from build123d import *

# Parameters (mm, degrees)
SKETCH2_W                = 45
SKETCH2_H                = 90
EXTRUDE2_DEPTH           = 9.525
SKETCH4_W                = 70
SKETCH4_H                = 9.525
CUT_EXTRUDE1_DEPTH       = 65.348470262
SKETCH5_W                = 8.5
SKETCH5_H                = 70
CUT_EXTRUDE2_DEPTH       = 54.797328001
FILLET1_R                = 6.35
F_6_0_6_DIAMETER_HOLE1_D = 6
M8_CLEARANCE_HOLE1_D     = 9


with BuildPart() as part:
    # Sketch2 → Extrude2 (new, symmetric)
    with BuildSketch(Plane(origin=(0, 0, 0), x_dir=(1, 0, 0), z_dir=(0, 1, 0))):
        Rectangle(SKETCH2_W, SKETCH2_H)
    extrude(amount=EXTRUDE2_DEPTH, both=True)

    # Sketch4 → Cut-Extrude1 (cut, through all)
    with BuildSketch(Plane(origin=(22.5, 0, 0), x_dir=(0, 0, -1), z_dir=(1, 0, 0))):
        with Locations((10, -4.7625)):
            Rectangle(SKETCH4_W, SKETCH4_H)
    extrude(amount=-CUT_EXTRUDE1_DEPTH, mode=Mode.SUBTRACT)

    # Sketch5 → Cut-Extrude2 (cut, through all)
    with BuildSketch(Plane(origin=(0, 9.525, 0), x_dir=(1, 0, 0), z_dir=(0, 1, 0))):
        with Locations((-18.25, 10)):
            Rectangle(SKETCH5_W, SKETCH5_H)
        with Locations((18.25, 10)):
            Rectangle(SKETCH5_W, SKETCH5_H)
    extrude(amount=-CUT_EXTRUDE2_DEPTH, mode=Mode.SUBTRACT)

    # Fillet1
    fillet1_edges = [part.edges().sort_by_distance(p)[0] for p in [
        (-14, 4.7625, 25),
        (14, 4.7625, 25),
    ]]
    fillet(fillet1_edges, radius=FILLET1_R)

    # Ø6.0 (6) Diameter Hole1 (through all)
    with Locations(Plane(origin=(0, 9.525, 0), x_dir=(-1, 0, 0), z_dir=(0, 1, 0))):
        with Locations((-8, -12.5), (8, -12.5)):
            Hole(F_6_0_6_DIAMETER_HOLE1_D / 2)

    # M8 Clearance Hole1 (through all)
    with Locations(Plane(origin=(0, 9.525, 0), x_dir=(-1, 0, 0), z_dir=(0, 1, 0))):
        with Locations((0, -27.5), (0, 2.5)):
            Hole(M8_CLEARANCE_HOLE1_D / 2)


solid = part.part
Geometry: final body of the model. Coordinates: model frame, mm. A direction names the side the tool comes from. Round coordinates to 2 decimals unless told otherwise and drop trailing zeros. Loops run counter-clockwise (first coordinate to the right, second up) from the corner with the lowest first, then second, coordinate; pieces in that order, holes last. Notation, with made-up numbers: M 44.5,46 L 94.5,46 A29 cw 94.5,80 Z; hole C 5,-20 d6. An arc over 180 degrees is marked long. One line per question, with ' | ' between items.
(1) Access query for faces 1 (the flat face through (-14, 5, -13)), 2 (the flat face through (14, 5, -13)), 3 (the flat face through (0, 0, -10)). Directions: +Z, -Z, +X, -X, +Y, -Y. A direction counts if a zero-diameter tool reaches every point of the face in a straight line with its end or side. Return the directions, or none.
Check result:
face 1: -Z, -X, +Y, -Y | face 2: -Z, +X, +Y, -Y | face 3: -Z, +X, -X, -Y
(2) Pull-direction query (Z, two-part tool) for faces 4 (the cylindrical face through (10.77, 4.7, -13.65)), 5 (the cylindrical face through (-15.81, 4.7, 23.09)), 6 (the flat face through (-22.5, 0, 35)); classes: +Z half, -Z half, draft (parallel to the pull), parting line (faces both ways), or undercut.
Check result:
face 4: undercut | face 5: -Z half | face 6: draft
(3) Cut plane A-A on x = 0. Return the cut outline in (y, z) (3 decimals).
Check result:
outline: M -9.525,25 L 0,25 L 0,7 L 9.525,7 L 9.525,45 L -9.525,45 Z; M 0,-45 L 9.525,-45 L 9.525,-32 L 0,-32 Z; M 0,-23 L 9.525,-23 L 9.525,-2 L 0,-2 Z
(4) Cut plane C-C on y = 2.25. Return the cut outline in (x, z), plus the area to 3 significant figures.
Check result:
outline: M -22.5,25 L -20.35,25 A6.35 cw -14,18.65 L -14,-45 L 14,-45 L 14,18.65 A6.35 cw 20.35,25 L 22.5,25 L 22.5,45 L -22.5,45 Z; hole C -8,-12.5 d6; hole C 0,-27.5 d9; hole C 0,2.5 d9; hole C 8,-12.5 d6 | area: 2,690 mm2
(5) Material intervals for line 1 along Z through (x, y) = (0, 2.5); line 2 along Z through (x, y) = (-8, 2.5); line 3 along Z through (x, y) = (1, 4.5), sorted ascending. Write a range as from..to.
Check result:
line 1: z = -45..-32, -23..-2, 7..45 | line 2: z = -45..-15.5, -9.5..45 | line 3: z = -45..-31.89, -23.11..-1.89, 6.89..45
(6) Cut plane B-B on z = -27.5. Return the cut outline in (x, y) (3 decimals).
Check result:
outline: M -14,0 L -4.5,0 L -4.5,9.525 L -14,9.525 Z; M 4.5,0 L 14,0 L 14,9.525 L 4.5,9.525 Z
(7) Contact query for flat-ended pins moving along their axis: P1, Ø11.5, axis at x = 0, z = 2.5, coming from the -Y side; P2, Ø3, axis at y = 3, z = -16.5, coming from the +X side; P3, Ø2, axis at y = 4, z = -17.5, coming from the -X side; P4, Ø3, axis at x = 16.5, z = -10.5, coming from the +Y side. Output: stop coordinate, or through.
Check result:
P1: stops at y = 0 | P2: stops at x = 14 | P3: stops at x = -14 | P4: passes through
(8) Cut plane D-D on x = -8. Return the cut outline in (y, z) (3 decimals).
Check result:
outline: M -9.525,25 L 0,25 L 0,-9.5 L 9.525,-9.5 L 9.525,45 L -9.525,45 Z; M 0,-45 L 9.525,-45 L 9.525,-15.5 L 0,-15.5 Z
